from build123d import *

# Parameters (mm, degrees)
CROQUIS1_R              = 5
SALIENTE_EXTRUIR1_DEPTH = 10
CROQUIS2_W              = 6
CROQUIS2_H              = 16
CORTAR_EXTRUIR1_DEPTH   = 16


with BuildPart() as part:
    # Croquis1 → Saliente-Extruir1 (new body)
    with BuildSketch(Plane.XY):
        with BuildLine():
            Line((-3.852526449, 10.48553719), (-2.852526449, 10.48553719))
            ThreePointArc((-2.852526449, 10.48553719), (2.097221019, 8.435284658), (4.147473551, 3.48553719))
            Line((4.147473551, 3.48553719), (4.147473551, -9.51446281))
            Line((4.147473551, -9.51446281), (-10.852526449, -9.51446281))
            Line((-10.852526449, -9.51446281), (-10.852526449, 3.48553719))
            ThreePointArc((-10.852526449, 3.48553719), (-8.802273917, 8.435284658), (-3.852526449, 10.48553719))
        make_face()
        with Locations((-3.352526449, 3.48553719)):
            Circle(CROQUIS1_R, mode=Mode.SUBTRACT)
    extrude(amount=SALIENTE_EXTRUIR1_DEPTH)

    # Croquis2 → Cortar-Extruir1 (cut, through all)
    with BuildSketch(Plane(origin=(4.147473551, 0, 0), x_dir=(0, 0, -1), z_dir=(1, 0, 0))):
        with Locations((-5, 2.48553719)):
            Rectangle(CROQUIS2_W, CROQUIS2_H)
    extrude(amount=-CORTAR_EXTRUIR1_DEPTH, mode=Mode.SUBTRACT)


solid = part.part
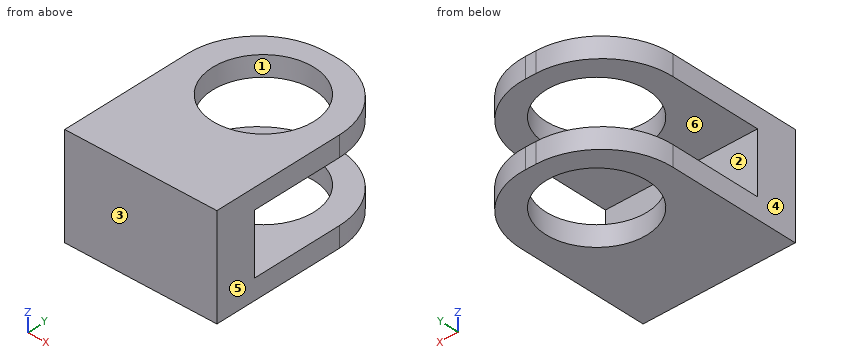
The listing builds one solid part. Answer for the finished solid, in the listing's coordinates (mm). Face numbers are marked on the shaded views. A direction names the side the tool comes from. Round coordinates to 2 decimals unless told otherwise and drop trailing zeros. Order: outer loops, then holes, each group sorted by start corner. A loop starts at its lowest first (then second) coordinate and runs counter-clockwise, first axis right, second up. Notation, with made-up numbers: (-3.75, -36.75) -> (43.25, -36.75) arc R12 cw to (43.25, -22.75) -> close; hole circle Ø11 at (77, 27). An arc over 180 degrees is marked (long way). Write each question's results on one line, items separated by ' | '. Start each with the question number.
Q1. Which of the six approach directions +Z, -Z, +X, -X, +Y, -Y give full straight-line access (tool end or side, diameter ignored) to the marked faces 5 and 6?
Q2. Find section D-D (y = 2). Determine the outline of the cut face in (x, z).
Q3. Find section B-B (x = -1). Determine the outline of the cut face in (y, z), then the cut area to 3 significant figures.
Q4. Find section A-A (y = -2.75). Determine the outline of the cut face in (x, z).
Q5. Straight lines are drawn through the part: probe 1 along Z at (x, y) = (-6.25, -1); probe 2 along X at (y, z) = (3.25, 9.5); probe 3 along X at (y, z) = (3.5, 8.75). For each, find the intervals that lie inside material, in ascending order. Write a range as from..to.
Q6. The mould has two halves that part along Y. Classify the marked faces 1, 2, 3 and 4: pulls with the +Y half, pulls with the -Y half, needs draft (parallel to the pull), parting line crosses it, or undercut.
Q7. Find section C-C (z = 8.25). Determine the outline of the cut face in (x, y), then the cut area to 3 significant figures.
Worked answers:
1) face 5: +Z, -Z, +X, +Y, -Y | face 6: +X, -X, +Y
2) outline: (-10.85, 0) -> (-8.13, 0) -> (-8.13, 2) -> (-10.85, 2) -> close; (-10.85, 8) -> (-8.13, 8) -> (-8.13, 10) -> (-10.85, 10) -> close; (1.42, 0) -> (4.15, 0) -> (4.15, 2) -> (1.42, 2) -> close; (1.42, 8) -> (4.15, 8) -> (4.15, 10) -> (1.42, 10) -> close
3) outline: (-9.51, 0) -> (-0.93, 0) -> (-0.93, 2) -> (-5.51, 2) -> (-5.51, 8) -> (-0.93, 8) -> (-0.93, 10) -> (-9.51, 10) -> close; (7.9, 0) -> (10.24, 0) -> (10.24, 2) -> (7.9, 2) -> close; (7.9, 8) -> (10.24, 8) -> (10.24, 10) -> (7.9, 10) -> close | area: 67.7 mm2
4) outline: (-10.85, 0) -> (4.15, 0) -> (4.15, 2) -> (-10.85, 2) -> close; (-10.85, 8) -> (4.15, 8) -> (4.15, 10) -> (-10.85, 10) -> close
5) probe 1: z = 0..2, 8..10 | probe 2: x = -10.85..-8.35, 1.64..4.15 | probe 3: x = -10.85..-8.35, 1.65..4.15
6) face 1: undercut | face 2: pulls with the +Y half | face 3: pulls with the -Y half | face 4: needs draft
7) outline: (-10.85, -9.51) -> (4.15, -9.51) -> (4.15, 3.49) arc R7 ccw to (-2.85, 10.49) -> (-3.85, 10.49) arc R7 ccw to (-10.85, 3.49) -> close; hole circle Ø10 at (-3.35, 3.49) | area: 200 mm2
